Autodesk Inventor part; units mm, degrees
ref_plane "YZ Plane" through (0, 0, 0) normal (1, 0, 0) x (0, 1, 0)
ref_plane "XZ Plane" through (0, 0, 0) normal (0, 1, 0) x (-1, 0, 0)
ref_plane "XY Plane" through (0, 0, 0) normal (0, 0, 1) x (1, 0, 0)
sketch "スケッチ1" plane through (0, 0, 0) normal (0, 0, 1) x (1, 0, 0)
  circle A0 centre (0, 0) radius 16.25
  line L0 (-25, 30.5) -> (25, 30.5)
  line L1 (25, 30.5) -> (25, -24.5)
  line L2 (25, -24.5) -> (-25, -24.5)
  line L3 (-25, -24.5) -> (-25, 30.5)
  line L4 (-25, -24.5) -> (-15, -24.5)
  line L5 (-15, -24.5) -> (-15, -30)
  line L6 (-15, -30) -> (-25, -30)
  line L7 (-25, -30) -> (-25, -24.5)
  line L8 (15, -24.5) -> (25, -24.5)
  line L9 (25, -24.5) -> (25, -30)
  line L10 (25, -30) -> (15, -30)
  line L11 (15, -30) -> (15, -24.5)
  circle A1 centre (0, 0) radius 25
  point P0 (0, 30.5)
  point P1 (-15, -24.5)
  point P2 (-25, 0)
  point P3 (25, 0)
  dimension "d0" = 32.5
  dimension "d1" = 24.5
  dimension "d2" = 50
  dimension "d3" = 55
  dimension "d6" = 5.5
  dimension "d7" = 10
extrude "押し出し1" add sketch "スケッチ1" along normal blind 5.5 contours A1 L2 L3 | A1 L2 | L1 L2 A1 | L2 L5 L6 L7 | L9 L10 L11 L2 picked at (-0.6529, -21.7105)
properties part number "motor_setter_front" material "木材 (カエデ材)"
Can you work these out from the model? Positions are in its coordinate system, mm. A direction names the side the tool comes from. Give positions to 0.01 mm unless a question says otherwise; leave off trailing zeros. Write each loop counter-clockwise with the first axis right and the second up, starting at its lowest first coordinate (ties: lowest second). Pieces come first, ordered by that corner, then holes. Notation, with made-up numbers: M -8.75,31 L 14.25,31 A22 ccw 14.25,44 Z; hole C 36.5,72.5 d1. An arc over 180 degrees is marked long. Answer in a Markdown table with one row per item. Add a question column.
Item 1: We'd pull the mould along X, two halves only. Please class faces 3 (the cylindrical face through (-0.55, 24.994, 2.712)), 4 (the flat face through (20, -30, 3)), 5 (the flat face through (0, -24.5, 3)): released by +X, released by -X, zero draft, split by the parting line, or undercut.
Item 2: Imagine slicing it at D-D, the plane x = 19.5. Write out the boundary of the cut face in (y, z).
Item 3: Imagine slicing it at B-B, the plane z = 1.6. Write out the boundary of the cut face in (x, y), plus the area to 3 significant figures.
Item 4: On a 3-axis mill with a long thin cutter (end or side, diameter ignored), from which of +Z, -Z, +X, -X, +Y, -Y can I reach the whole of each face in a straight line? I mean faces 1 (the flat face through (15, -27, 3)), 2 (the flat face through (-25, -15, 3)). Say none if no direction works.
Item 5: Imagine slicing it at A-A, the plane x = 0. Write out the boundary of the cut face in (y, z), plus the area to 3 significant figures.
Item 6: Please list where these lines run through material, in increasing order: L1, parallel to Y at x = 0, z = 2.65; L2, parallel to X at y = -26.5, z = 5; L3, parallel to Y at x = 8, z = 0.45.
Item 7: Imagine slicing it at C-C, the plane y = 12. Write out the boundary of the cut face in (x, z), plus the area to 3 significant figures.
Evaluation:
| question | item | result |
|---|---|---|
| 1 | face 3 | split by the parting line |
| 1 | face 4 | zero draft |
| 1 | face 5 | undercut |
| 2 | outline | M -30,0 L 15.64,0 L 15.64,5.5 L -30,5.5 Z |
| 3 | outline | M -25,-30 L -15,-30 L -15,-24.5 L 15,-24.5 L 15,-30 L 25,-30 L 25,0 A25 ccw -25,0 Z; hole C 0,0 d32.5 |
| 3 | area | 1,490 mm² |
| 4 | face 1 | +Z, -Z, -Y |
| 4 | face 2 | +Z, -Z, -X, +Y, -Y |
| 5 | outline | M -24.5,0 L -16.25,0 L -16.25,5.5 L -24.5,5.5 Z; M 16.25,0 L 25,0 L 25,5.5 L 16.25,5.5 Z |
| 5 | area | 93.5 mm² |
| 6 | L1 | y = -24.5 to -16.25, 16.25 to 25 |
| 6 | L2 | x = -25 to -15, 15 to 25 |
| 6 | L3 | y = -24.5 to -14.14, 14.14 to 23.69 |
| 7 | outline | M -21.93,0 L -10.96,0 L -10.96,5.5 L -21.93,5.5 Z; M 10.96,0 L 21.93,0 L 21.93,5.5 L 10.96,5.5 Z |
| 7 | area | 121 mm² |
